Autodesk Inventor part; units mm, degrees
ref_plane "Work Plane1" through (0.75, 1.7337, 0.1) normal (0, 0, 1) x (1, 0, 0)
ref_plane "YZ Plane" through (0, 0, 0) normal (1, 0, 0) x (0, 1, 0)
ref_plane "XZ Plane" through (0, 0, 0) normal (0, 1, 0) x (-1, 0, 0)
ref_plane "Work Plane1" through (0.75, 1.7337, 0.1) normal (0, 0, 1) x (1, 0, 0)
sketch "Sketch1" plane through (0.75, 1.7337, 0.1) normal (0, 0, 1) x (1, 0, 0)
  line L0 (14.9531, -9.2968) -> (14.9531, -22.3927)
  line L1 (14.9531, -9.2968) -> (11.1531, -9.2968)
  line L2 (-21.9469, -8.1274) -> (-21.9469, -20.8182)
  line L3 (-21.9469, -20.8182) -> (-17.7469, -20.8182)
  line L4 (10.3531, -18.6448) -> (-17.3469, -18.6448)
  line L5 (-17.3469, -18.6448) -> (-17.3469, -17.8448)
  line L6 (-17.3469, -17.8448) -> (10.3531, -17.8448)
  line L7 (10.3531, -17.8448) -> (10.3531, -18.6448)
  line L8 (14.9531, -22.3927) -> (10.7531, -22.3927)
  circle A0 centre (12.7531, -12.5861) radius 2
  circle A1 centre (12.7531, -12.5861) radius 2
  circle A2 centre (12.7531, -19.134) radius 2
  circle A3 centre (12.7531, -19.134) radius 2
  line L9 (11.1531, -10.0071) -> (11.1531, -9.2968)
  line L10 (11.1531, -10.0071) -> (10.7531, -10.0071)
  line L11 (10.7531, -12.5861) -> (10.7531, -10.0071)
  line L12 (10.7531, -19.134) -> (10.7531, -12.5861)
  line L13 (10.7531, -22.3927) -> (10.7531, -19.134)
  line L14 (-17.7469, -8.1274) -> (-17.7469, -20.8182)
  line L15 (-21.9469, -8.1274) -> (-17.7469, -8.1274)
  ellipse E0 centre (-19.8469, -17.6455) end of major axis (-21.8469, -17.6455) minor radius 1.9381
  ellipse E1 centre (-19.8469, -11.3001) end of major axis (-21.8469, -11.3001) minor radius 1.9381
  point P0 (-0.75, -1.7337)
  point P1 (-18.5469, -9.3259)
  dimension "d2" = 0.8
extrude "Extrusion1" add sketch "Sketch1" along normal blind 20.9 and the other way blind 0.7 contours L4 L5 L6 L7
sketch "Sketch3" plane through (-16.5969, -16.911, -0.6) normal (0, -1, 0) x (1, 0, 0)
  line L0 (27.7, 0) -> (0, 0)
  line L1 (27.7, 0) -> (27.7, 21.6)
  line L2 (0, 21.6) -> (27.7, 21.6)
  line L3 (0, 0) -> (0, 21.6)
  circle A0 centre (24.95, 18.85) radius 2.75
  circle A1 centre (2.75, 18.85) radius 2.75
  line L4 (27.7, 21.6) -> (27.7, 0)
  line L5 (0, 0) -> (0, 21.6)
  point P0 (16.5969, 0.6)
  dimension "d17" = 5.5
  dimension "d18" = 5.5
  dimension "d19" = 0
  dimension "d20" = 0
hole "Hole1" at (8.3531, -16.911, 18.25) at (-13.8469, -16.911, 18.25) direction (0, 1, 0) diameter 2.5 end through all
fillet "Fillet1" radius 1 4 edges at (11.1031, -16.511, -0.6) (-16.5969, -16.511, -0.6) (-16.5969, -16.511, 21) (11.1031, -16.511, 21)
properties part number "PCB_Controller"
Can you work these out from the model? Positions are in its coordinate system, mm. Round coordinates to 2 decimals unless told otherwise and drop trailing zeros. Loops run counter-clockwise (first coordinate to the right, second up) from the corner with the lowest first, then second, coordinate; pieces in that order, holes last. Notation, with made-up numbers: (24.25, 30.25) - (54.25, 30.25) arc R7 cw to (54.25, 38.25) - close; hole circle Ø7 at (22, 69). An arc over 180 degrees is marked (long way). Answer in a Markdown table with one row per item. Add a question column.
Q1. I want a section at B-B on y = -16.7. List the corners of the cut face in (x, z) for me.
Q2. I need wall thicknesses on L1, parallel to X at y = -16.7, z = 18.25; L2, parallel to X at y = -16.5, z = 17.75; L3, parallel to Z at x = -13.5, y = -16.4. Which ranges of each line are inside material? Lowest first, please.
Q3. We'd pull the mould along X, two halves only. Please class faces 1 (the cylindrical face through (7.3, -16.51, 17.58)), 2 (the flat face through (-2.9, -16.5, -0.6)), 3 (the cylindrical face through (-16.31, -16.51, 20.7)): pulls with the +X half, pulls with the -X half, needs draft (parallel to the pull), parting line crosses it, or undercut.
Q4. I want a section at A-A on z = 18.25. List the corners of the cut face in (x, y) for me.
A:
| question | item | result |
|---|---|---|
| 1 | outline | (-16.6, 0.4) arc R1 ccw to (-15.6, -0.6) - (10.1, -0.6) arc R1 ccw to (11.1, 0.4) - (11.1, 20) arc R1 ccw to (10.1, 21) - (-15.6, 21) arc R1 ccw to (-16.6, 20) - close; hole circle Ø2.5 at (-13.85, 18.25); hole circle Ø2.5 at (8.35, 18.25) |
| 2 | L1 | -16.6 to -15.1, -12.6 to 7.1, 9.6 to 11.1 |
| 2 | L2 | -16.6 to -14.99, -12.7 to 7.21, 9.5 to 11.1 |
| 2 | L3 | -0.6 to 17.05, 19.45 to 21 |
| 3 | face 1 | undercut |
| 3 | face 2 | needs draft |
| 3 | face 3 | pulls with the -X half |
| 4 | outline | (-16.6, -16.91) - (-15.1, -16.91) - (-15.1, -16.11) - (-16.6, -16.11) - close; (-12.6, -16.91) - (7.1, -16.91) - (7.1, -16.11) - (-12.6, -16.11) - close; (9.6, -16.91) - (11.1, -16.91) - (11.1, -16.11) - (9.6, -16.11) - close |
